Read the model definition and answer for the solid it produces. Units are mm, in the model's axes. A direction names the side the tool comes from. Coordinates: 2 decimals unless noted, no trailing zeros. Write each loop counter-clockwise with the first axis right and the second up, starting at its lowest first coordinate (ties: lowest second). Pieces come first, ordered by that corner, then holes. Notation, with made-up numbers: (10, 61) -> (20, 61) arc R33 cw to (20, 94) -> close; hole circle Ø7 at (-2, 10). An arc over 180 degrees is marked (long way). Return JSON: item names as keys, results as strings.
from build123d import *

# Parameters (mm, degrees)
SKETCH_1_W      = 10
SKETCH_1_H      = 12
SKETCH_1_R      = 1.5
SKETCH_1_R_2    = 0.8
SKETCH_1_R_3    = 0.7
EXTRUDE_1_DEPTH = 9
SKETCH_2_R      = 2
SKETCH_2_R_2    = 1.5
EXTRUDE_2_DEPTH = 0.7
FILLET_1_R      = 1


with BuildPart() as part:
    # 草图1 → 凸台-拉伸1 (new body)
    with BuildSketch(Plane.XY):
        Rectangle(SKETCH_1_W, SKETCH_1_H)
        Circle(SKETCH_1_R, mode=Mode.SUBTRACT)
        with Locations((0, 4.5)):
            Circle(SKETCH_1_R_2, mode=Mode.SUBTRACT)
        with Locations(Location((0, -4.5, 0), (0, 0, 180))):
            Circle(SKETCH_1_R_2, mode=Mode.SUBTRACT)
        with Locations((-3, 4)):
            Circle(SKETCH_1_R_3, mode=Mode.SUBTRACT)
        with Locations((3, -4)):
            Circle(SKETCH_1_R_3, mode=Mode.SUBTRACT)
    extrude(amount=EXTRUDE_1_DEPTH)

    # 草图2 → 凸台-拉伸2 (add)
    with BuildSketch(Plane.XY.offset(9)):
        with Locations(Location((0, 0, 0), (0, 0, 180))):
            Circle(SKETCH_2_R)
        Circle(SKETCH_2_R_2, mode=Mode.SUBTRACT)
    extrude(amount=EXTRUDE_2_DEPTH)

    # 圆角1
    fillet_1_edges = [part.edges().sort_by_distance(p)[0] for p in [
        (5, -6, 4.5),
        (-5, -6, 4.5),
        (-5, 6, 4.5),
        (5, 6, 4.5),
    ]]
    fillet(fillet_1_edges, radius=FILLET_1_R)


solid = part.part
1. The part is cut by section D-D (z = 5.5). Determine the outline of the cut face in (x, y).
Taken from the geometry:
{"outline": "(-5, -5) arc R1 ccw to (-4, -6) -> (4, -6) arc R1 ccw to (5, -5) -> (5, 5) arc R1 ccw to (4, 6) -> (-4, 6) arc R1 ccw to (-5, 5) -> close; hole circle Ø1.4 at (-3, 4); hole circle Ø3 at (0, 0); hole circle Ø1.6 at (0, -4.5); hole circle Ø1.6 at (0, 4.5); hole circle Ø1.4 at (3, -4)"}
2. The part is cut by section C-C (y = -0.25). Determine the outline of the cut face in (x, z).
Taken from the geometry:
{"outline": "(-5, 0) -> (-1.48, 0) -> (-1.48, 9.7) -> (-1.98, 9.7) -> (-1.98, 9) -> (-5, 9) -> close; (1.48, 0) -> (5, 0) -> (5, 9) -> (1.98, 9) -> (1.98, 9.7) -> (1.48, 9.7) -> close"}
3. A tool of negligible diameter and unlimited length cuts with its end or side. For faces 4 (the face through (0.434, 1.952, 9.345)), 5 (the face through (4.715, -5.699, 4.563)), from which of +Z, -Z, +X, -X, +Y, -Y can it reach the whole face along a straight path? Write none if from no direction.
Taken from the geometry:
{"face 4": "+Z", "face 5": "+Z, -Z, +X, -Y"}
4. The part is cut by section B-B (x = -3). Determine the outline of the cut face in (y, z), then the cut area to 3 significant figures.
Taken from the geometry:
{"outline": "(-6, 0) -> (3.3, 0) -> (3.3, 9) -> (-6, 9) -> close; (4.7, 0) -> (6, 0) -> (6, 9) -> (4.7, 9) -> close", "area": "95.4 mm2"}
5. Flat-ended cylindrical pins translate along their axes: pin 1 Ø1 at (x, y) = (-1.5, 4) entering from +Z; pin 2 Ø6 at (x, y) = (1, -2.5) entering from +Z. Find the tip coordinate at first contact, or state that the pin passes through.
Taken from the geometry:
{"pin 1": "stops at z = 9", "pin 2": "stops at z = 9.7"}
6. For a pull along X with two mould halves and no side action, classify faces 1 (the face through (4.715, 5.699, 4.563)), 2 (the face through (0, -6, 4)), 3 (the face through (0.17, -3.72, 4.44)) as +X half, -X half, draft (parallel to the pull), parting line (faces both ways), or undercut.
Taken from the geometry:
{"face 1": "+X half", "face 2": "draft", "face 3": "undercut"}
7. Consider L1, parallel to Y at x = 0, z = 8.5; L2, parallel to Y at x = -3, z = 0.5; L3, parallel to Z at x = 3.5, y = -3. Determine where each line is inside the solid, lowest interval first.
Taken from the geometry:
{"L1": "y = -6 to -5.3, -3.7 to -1.5, 1.5 to 3.7, 5.3 to 6", "L2": "y = -6 to 3.3, 4.7 to 6", "L3": "z = 0 to 9"}
8. The part is cut by section A-A (x = 0). Determine the outline of the cut face in (y, z).
Taken from the geometry:
{"outline": "(-6, 0) -> (-5.3, 0) -> (-5.3, 9) -> (-6, 9) -> close; (-3.7, 0) -> (-1.5, 0) -> (-1.5, 9.7) -> (-2, 9.7) -> (-2, 9) -> (-3.7, 9) -> close; (1.5, 0) -> (3.7, 0) -> (3.7, 9) -> (2, 9) -> (2, 9.7) -> (1.5, 9.7) -> close; (5.3, 0) -> (6, 0) -> (6, 9) -> (5.3, 9) -> close"}
